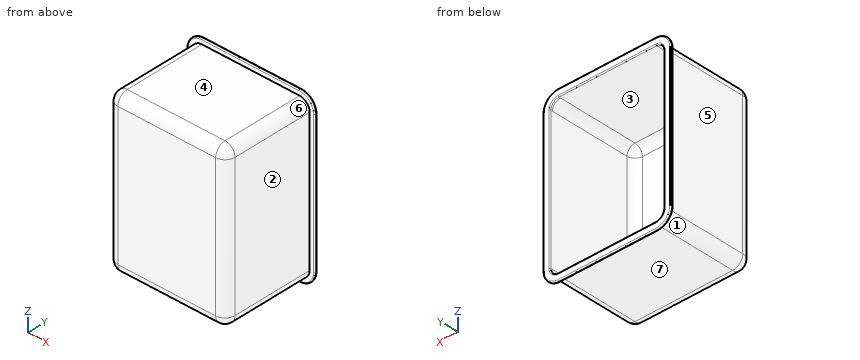
```python
from build123d import *

# Parameters (mm, degrees)
SKETCH1_W           = 149.352
SKETCH1_H           = 203.2
BOSS_EXTRUDE1_DEPTH = 114.3
FILLET1_R           = 12.7
SHELL1_T            = -2.54
BOSS_EXTRUDE2_START = 3.175
BOSS_EXTRUDE2_DEPTH = 3.175
FILLET2_R           = 1.27


with BuildPart() as part:
    # Sketch1 → Boss-Extrude1 (new body)
    with BuildSketch(Plane(origin=(0, 0, 0), x_dir=(1, 0, 0), z_dir=(0, 1, 0))):
        Rectangle(SKETCH1_W, SKETCH1_H)
    extrude(amount=BOSS_EXTRUDE1_DEPTH)

    # Fillet1
    fillet1_edges = [part.edges().sort_by_distance(p)[0] for p in [
        (0, 0, 101.6),
        (-74.676, 0, 0),
        (0, 0, -101.6),
        (74.676, 0, 0),
        (74.676, 57.15, 101.6),
        (-74.676, 57.15, 101.6),
        (-74.676, 57.15, -101.6),
        (74.676, 57.15, -101.6),
    ]]
    fillet(fillet1_edges, radius=FILLET1_R)

    # Shell1
    shell1_openings = [part.faces().sort_by_distance(p)[0] for p in [
        (0, 114.3, 0),
    ]]
    offset(amount=SHELL1_T, openings=shell1_openings, kind=Kind.INTERSECTION)

    # Sketch2 → Boss-Extrude2 (add)
    with BuildSketch(Plane(origin=(0, 114.3, 0), x_dir=(1, 0, 0), z_dir=(0, 1, 0)).offset(BOSS_EXTRUDE2_START)):
        with BuildLine():
            Line((61.976, 107.95), (-61.976, 107.95))
            ThreePointArc((-61.976, 107.95), (-75.446384182, 102.370384182), (-81.026, 88.9))
            Line((-81.026, 88.9), (-81.026, -88.9))
            ThreePointArc((-81.026, -88.9), (-75.446384182, -102.370384182), (-61.976, -107.95))
            Line((-61.976, -107.95), (61.976, -107.95))
            ThreePointArc((61.976, -107.95), (75.446384182, -102.370384182), (81.026, -88.9))
            Line((81.026, -88.9), (81.026, 88.9))
            ThreePointArc((81.026, 88.9), (75.446384182, 102.370384182), (61.976, 107.95))
        make_face()
        with BuildLine():
            Line((-72.136, 88.9), (-72.136, -88.9))
            ThreePointArc((-72.136, -88.9), (-69.160204897, -96.084204897), (-61.976, -99.06))
            Line((-61.976, -99.06), (61.976, -99.06))
            ThreePointArc((61.976, -99.06), (69.160204897, -96.084204897), (72.136, -88.9))
            Line((72.136, -88.9), (72.136, 88.9))
            ThreePointArc((72.136, 88.9), (69.160204897, 96.084204897), (61.976, 99.06))
            Line((61.976, 99.06), (-61.976, 99.06))
            ThreePointArc((-61.976, 99.06), (-69.160204897, 96.084204897), (-72.136, 88.9))
        make_face(mode=Mode.SUBTRACT)
    extrude(amount=-BOSS_EXTRUDE2_DEPTH)

    # Fillet2
    fillet2_edges = [part.edges().sort_by_distance(p)[0] for p in [
        (75.446384182, 117.475, -102.370384182),
        (0, 117.475, -107.95),
        (-75.446384182, 117.475, -102.370384182),
        (-81.026, 117.475, 0),
        (-75.446384182, 117.475, 102.370384182),
        (0, 117.475, 107.95),
        (75.446384182, 117.475, 102.370384182),
        (81.026, 117.475, 0),
        (75.446384182, 114.3, -102.370384182),
        (0, 114.3, -107.95),
        (-75.446384182, 114.3, -102.370384182),
        (-81.026, 114.3, 0),
        (-75.446384182, 114.3, 102.370384182),
        (0, 114.3, 107.95),
        (75.446384182, 114.3, 102.370384182),
        (81.026, 114.3, 0),
        (-69.160204897, 117.475, -96.084204897),
        (-72.136, 117.475, 0),
        (-69.160204897, 117.475, 96.084204897),
        (0, 117.475, 99.06),
        (69.160204897, 117.475, 96.084204897),
        (72.136, 117.475, 0),
        (69.160204897, 117.475, -96.084204897),
        (0, 117.475, -99.06),
    ]]
    fillet(fillet2_edges, radius=FILLET2_R)


solid = part.part
```
Input: part model. Units: mm. Frame: model coordinates. Face numbers are marked on the shaded views. A direction names the side the tool comes from. Give positions to 0.01 mm unless a question says otherwise; leave off trailing zeros. Order: outer loops, then holes, each group sorted by start corner. A loop starts at its lowest first (then second) coordinate and runs counter-clockwise, first axis right, second up. Notation, with made-up numbers: (49.5, -31) - (54.5, -31) arc R23 cw to (54.5, -22) - close; hole circle Ø1 at (17, 26.25). An arc over 180 degrees is marked (long way). Use a Markdown table: item, result.
(1) Draft query along Z for the marked faces 1, 2 and 3. Return one class per face: released by +Z, released by -Z, zero draft, split by the parting line, or undercut.
Computed values:
| item | result |
|---|---|
| face 1 | released by -Z |
| face 2 | zero draft |
| face 3 | undercut |
(2) Pin query (flat end, axial travel): pin 1 (3 mm diameter, centred on y = 18.5, z = -85, fed in from +X); pin 2 (5 mm diameter, centred on x = -6, y = 65.5, fed in from -Z); pin 3 (8 mm diameter, centred on x = 24, z = -28.5, fed in from +Y). Return the tip coordinate at first contact, or that it passes through.
Computed values:
| item | result |
|---|---|
| pin 1 | stops at x = 74.68 |
| pin 2 | stops at z = -101.6 |
| pin 3 | stops at y = 2.54 |
(3) Access query for the marked faces 4, 5, 6 and 7. Directions: +Z, -Z, +X, -X, +Y, -Y. A direction counts if a zero-diameter tool reaches every point of the face in a straight line with its end or side. Return the directions, or none.
Computed values:
| item | result |
|---|---|
| face 4 | +Z, +X, -X, -Y |
| face 5 | +Z, -Z, -X, -Y |
| face 6 | +Z, +X, -Y |
| face 7 | -Z, +X, -X, -Y |
(4) Section query B-B (z = -60.5). Output: boundary loops of the cut face in (x, y) (3 decimals), then the cut area to 3 significant figures.
Computed values:
| item | result |
|---|---|
| outline | (-81.026, 115.57) arc R1.27 ccw to (-79.756, 114.3) - (-74.676, 114.3) - (-74.676, 12.7) arc R12.7 ccw to (-61.976, 0) - (61.976, 0) arc R12.7 ccw to (74.676, 12.7) - (74.676, 114.3) - (79.756, 114.3) arc R1.27 ccw to (81.026, 115.57) - (81.026, 116.205) arc R1.27 ccw to (79.756, 117.475) - (73.406, 117.475) arc R1.27 ccw to (72.136, 116.205) - (72.136, 12.7) arc R10.16 cw to (61.976, 2.54) - (-61.976, 2.54) arc R10.16 cw to (-72.136, 12.7) - (-72.136, 116.205) arc R1.27 ccw to (-73.406, 117.475) - (-79.756, 117.475) arc R1.27 ccw to (-81.026, 116.205) - close |
| area | 977 mm2 |
(5) Section query A-A (y = 73). Output: boundary loops of the cut face in (x, z).
Computed values:
| item | result |
|---|---|
| outline | (-74.68, -88.9) arc R12.7 ccw to (-61.98, -101.6) - (61.98, -101.6) arc R12.7 ccw to (74.68, -88.9) - (74.68, 88.9) arc R12.7 ccw to (61.98, 101.6) - (-61.98, 101.6) arc R12.7 ccw to (-74.68, 88.9) - close; hole (-72.14, -88.9) arc R10.16 ccw to (-61.98, -99.06) - (61.98, -99.06) arc R10.16 ccw to (72.14, -88.9) - (72.14, 88.9) arc R10.16 ccw to (61.98, 99.06) - (-61.98, 99.06) arc R10.16 ccw to (-72.14, 88.9) - close |
(6) Section query C-C (x = -9). Output: boundary loops of the cut face in (y, z) (3 decimals), then the cut area to 3 significant figures.
Computed values:
| item | result |
|---|---|
| outline | (0, -88.9) arc R12.7 ccw to (12.7, -101.6) - (114.3, -101.6) - (114.3, -106.68) arc R1.27 ccw to (115.57, -107.95) - (116.205, -107.95) arc R1.27 ccw to (117.475, -106.68) - (117.475, -100.33) arc R1.27 ccw to (116.205, -99.06) - (12.7, -99.06) arc R10.16 cw to (2.54, -88.9) - (2.54, 88.9) arc R10.16 cw to (12.7, 99.06) - (116.205, 99.06) arc R1.27 ccw to (117.475, 100.33) - (117.475, 106.68) arc R1.27 ccw to (116.205, 107.95) - (115.57, 107.95) arc R1.27 ccw to (114.3, 106.68) - (114.3, 101.6) - (12.7, 101.6) arc R12.7 ccw to (0, 88.9) - close |
| area | 1,110 mm2 |
(7) Line query: line 1 (Z direction, x = 57.5, y = 46.5); line 2 (X direction, y = 42.5, z = -58.5); line 3 (X direction, y = 9, z = -13.5). Output: solid intervals per line, ascending. Write a range as from..to.
Computed values:
| item | result |
|---|---|
| line 1 | z = -101.6..-99.06, 99.06..101.6 |
| line 2 | x = -74.68..-72.14, 72.14..74.68 |
| line 3 | x = -74.13..-71.44, 71.44..74.13 |
